Could you check a few things on this model? Use its own coordinates, in mm. Give positions to 0.01 mm unless a question says otherwise; leave off trailing zeros. Order: outer loops, then holes, each group sorted by start corner. A loop starts at its lowest first (then second) coordinate and runs counter-clockwise, first axis right, second up. Notation, with made-up numbers: M 84.5,-14 L 104.5,-14 A17 cw 104.5,-7 Z; hole C 54.5,48 d9. An arc over 180 degrees is marked long. Use a Markdown table: item, result. Add a question column.
Item 1: Suppose I cut it at A-A on y = 5.5. Count the separate pieces of the cut face and the enclosed holes in it, plus the area to 3 significant figures.
Item 2: I'm going to push flat-ended pins straight in: pin 1 Ø6 at (x, z) = (28, 75) entering from -Y; pin 2 Ø2 at (y, z) = (4.5, 161) entering from +X; pin 3 Ø1 at (y, z) = (8.5, -76) entering from -X; pin 4 Ø2 at (x, y) = (110, 6.5) entering from +Z. Where does each tip first touch, or does it pass through?
Item 3: Suppose I cut it at C-C on z = 130. Write out the boundary of the cut face in (x, y), plus the area to 3 significant figures.
Item 4: If I drill on L1, parallel to Z at x = 0, y = 5.75; L2, parallel to X at y = 7.25, z = 105.5; L3, parallel to Z at x = -188, y = 5.75, over which ranges is the centre line in solid material (lowest first)? Write a range as from..to.
Item 5: Suppose I cut it at B-B on x = 195.5. Write out the boundary of the cut face in (y, z).
Autodesk Inventor part; units mm, degrees
ref_plane "YZ Plane" through (0, 0, 0) normal (1, 0, 0) x (0, 1, 0)
ref_plane "XZ Plane" through (0, 0, 0) normal (0, 1, 0) x (-1, 0, 0)
ref_plane "XY Plane" through (0, 0, 0) normal (0, 0, 1) x (1, 0, 0)
sketch "Sketch1" plane through (0, 0, 0) normal (0, 1, 0) x (-1, 0, 0)
  arc A0 (-195.1682, -43.6963) -> (-195.1682, -43.6963) centre (0, 0) ccw construction
  spline S0 degree 3 poles (212.7614, 63.8524) (213.1534, 65.8524) (213.5259, 67.8561) (213.8787, 69.8633) knots 0 0 0 0 0.019635 0.019635 0.019635 0.019635 construction
  circle A1 centre (0, 0) radius 225
  line L0 (0, 0) -> (0, 120) construction
  line L1 (0, 0) -> (0, -120) construction
  line L2 (0, 0) -> (-120, 0) construction
  line L3 (0, 0) -> (120, 0) construction
  circle A2 centre (-120, 0) radius 3.5
  circle A3 centre (0, -120) radius 3.5
  circle A4 centre (120, 0) radius 3.5
  circle A5 centre (0, 120) radius 3.5
  circle A6 centre (0, -211.1656) radius 4
  circle A7 centre (105.5828, -182.8748) radius 4
  circle A8 centre (182.8748, -105.5828) radius 4
  circle A9 centre (211.1656, 0) radius 4
  circle A10 centre (182.8748, 105.5828) radius 4
  circle A11 centre (105.5828, 182.8748) radius 4
  circle A12 centre (0, 211.1656) radius 4
  circle A13 centre (-105.5828, 182.8748) radius 4
  circle A14 centre (-182.8748, 105.5828) radius 4
  circle A15 centre (-211.1656, 0) radius 4
  circle A16 centre (-182.8748, -105.5828) radius 4
  circle A17 centre (-105.5828, -182.8748) radius 4
  circle A18 centre (225, 0) radius 25
  line L4 (225, 0) -> (242.9975, 17.352)
  line L5 (225, 0) -> (250, 0)
  arc A19 (217.6933, 56.8737) -> (242.9975, 17.352) centre (295.1945, 78.633) ccw
  arc A20 (242.9975, -17.352) -> (217.6933, -56.8737) centre (295.1945, -78.633) ccw
  point P0 (217.6933, -56.8737)
  point P1 (242.9975, -17.352)
  dimension "d0" = 120
  dimension "d1" = 120
  dimension "d2" = 120
  dimension "d3" = 120
  dimension "d4" = 7
  dimension "d5" = 7
  dimension "d6" = 7
  dimension "d7" = 7
  dimension "d10" = 450
  dimension "d11" = 8
  dimension "d14" = 360
  dimension "d16" = 50
  dimension "d17" = 43.954
extrude "Extrusion1" add sketch "Sketch1" along normal blind 10 contours A1 A18 | A19 A18 A1 | A1 A18 A20 | A18 A19 L4 A1 | A1 A18 | A1 L5 A18 A20 | L4 A18 L5
properties part number "MDF Board"
Findings below:
| question | item | result |
|---|---|---|
| 1 | separate pieces | 1 |
| 1 | enclosed holes | 16 |
| 1 | area | 160,000 mm^2 |
| 2 | pin 1 | stops at y = 0 |
| 2 | pin 2 | stops at x = 158.19 |
| 2 | pin 3 | stops at x = -211.95 |
| 2 | pin 4 | stops at z = 196.83 |
| 3 | outline | M -183.64,0 L 183.64,0 L 183.64,10 L -183.64,10 Z |
| 3 | area | 3,670 mm^2 |
| 4 | L1 | z = -225..-215.17, -207.17..-123.5, -116.5..116.5, 123.5..207.17, 215.17..225 |
| 4 | L2 | x = -198.73..-186.87, -178.88..178.88, 186.87..198.73 |
| 4 | L3 | z = -123.62..123.62 |
| 5 | outline | M 0,-111.38 L 10,-111.38 L 10,111.38 L 0,111.38 Z |
